Autodesk Inventor part; units mm, degrees
ref_plane "YZ Plane" through (0, 0, 0) normal (1, 0, 0) x (0, 1, 0)
ref_plane "XZ Plane" through (0, 0, 0) normal (0, 1, 0) x (-1, 0, 0)
ref_plane "XY Plane" through (0, 0, 0) normal (0, 0, 1) x (1, 0, 0)
sketch "Sketch1" plane through (0, 0, 0) normal (0, 1, 0) x (-1, 0, 0)
  line L0 (-27.5, 44) -> (27.5, 44)
  line L1 (27.5, 44) -> (27.5, -44)
  line L2 (27.5, -44) -> (-27.5, -44)
  line L3 (-27.5, -44) -> (-27.5, 44)
  line L4 (-27.5, 44) -> (27.5, -44) construction
  line L5 (27.5, 44) -> (-27.5, -44) construction
  line L6 (-27.5, 44) -> (-22.5, 44)
  line L7 (-22.5, 44) -> (-22.5, 35)
  line L8 (-22.5, 35) -> (-27.5, 35)
  line L9 (-27.5, 35) -> (-27.5, 44)
  line L10 (-22.5, 35) -> (-17.5, 35)
  line L11 (-17.5, 35) -> (-17.5, 30)
  line L12 (-17.5, 30) -> (-22.5, 30)
  line L13 (-22.5, 30) -> (-22.5, 35)
  line L14 (-17.5, 30) -> (-12.5, 30)
  line L15 (-12.5, 30) -> (-12.5, 25)
  line L16 (-12.5, 25) -> (-17.5, 25)
  line L17 (-17.5, 25) -> (-17.5, 30)
  line L18 (-12.5, 25) -> (-7.5, 25)
  line L19 (-7.5, 25) -> (-7.5, 20)
  line L20 (-7.5, 20) -> (-12.5, 20)
  line L21 (-12.5, 20) -> (-12.5, 25)
  line L22 (-7.5, 20) -> (-2.5, 20)
  line L23 (-2.5, 20) -> (-2.5, 15)
  line L24 (-2.5, 15) -> (-7.5, 15)
  line L25 (-7.5, 15) -> (-7.5, 20)
  line L26 (-2.5, 15) -> (2.5, 15)
  line L27 (2.5, 15) -> (2.5, 10)
  line L28 (2.5, 10) -> (-2.5, 10)
  line L29 (-2.5, 10) -> (-2.5, 15)
  line L30 (2.5, 10) -> (7.5, 10)
  line L31 (7.5, 10) -> (7.5, 5)
  line L32 (7.5, 5) -> (2.5, 5)
  line L33 (2.5, 5) -> (2.5, 10)
  line L34 (13, 5) -> (13, 0)
  line L35 (13, 0) -> (8, 0)
  line L36 (8, 0) -> (8, 5)
  line L37 (-27.5, -44) -> (27.5, 44) construction
  line L38 (-22.5, -35) -> (-27.5, -35)
  line L39 (-17.5, -30) -> (-22.5, -30)
  line L40 (-22.5, -30) -> (-22.5, -35)
  line L41 (-17.5, -25) -> (-17.5, -30)
  line L42 (-7.5, -20) -> (-12.5, -20)
  line L43 (-12.5, -20) -> (-12.5, -25)
  line L44 (-2.5, -15) -> (-7.5, -15)
  line L45 (-7.5, -15) -> (-7.5, -20)
  line L46 (2.5, -10) -> (-2.5, -10)
  line L47 (-2.5, -10) -> (-2.5, -15)
  line L48 (7.5, -5) -> (2.5, -5)
  line L49 (2.5, -5) -> (2.5, -10)
  line L50 (8, 0) -> (8, -5)
  line L51 (7.5, 5) -> (7.5, -5)
  line L52 (27.5, 0) -> (21.5, 0)
  circle A0 centre (21.5, 0) radius 6
  line L53 (-12.5, -25) -> (-17.5, -25)
  point P0 (0, 0)
  dimension "d0" = 55
  dimension "d1" = 88
  dimension "d2" = 5
  dimension "d3" = 9
  dimension "d4" = 5
  dimension "d5" = 5
  dimension "d6" = 5
  dimension "d7" = 5
  dimension "d8" = 5
  dimension "d9" = 5
  dimension "d10" = 5
  dimension "d11" = 5
  dimension "d12" = 5
  dimension "d13" = 5
  dimension "d14" = 5
  dimension "d15" = 5
  dimension "d16" = 5
  dimension "d17" = 5
  dimension "d18" = 6
extrude "Extrusion1" add sketch "Sketch1" along normal blind 20 contours L0 L7 L8 L3 | A0 | L0 L1 L2 L3 L38 L40 L39 L41 L53 L43 L42 L45 L44 L47 L46 L49 L48 L51 L31 L30 L27 L26 L23 L22 L19 L18 L15 L14 L11 L10 L7 | L10 L11 L12 L13 | L14 L15 L16 L17 | L18 L19 L20 L21 | L22 L23 L24 L25 | L26 L27 L28 L29 | L30 L31 L32 L33
sketch "Sketch2" plane through (0, 0, 0) normal (0, -1, 0) x (1, 0, 0)
  line L0 (-27.5, -44) -> (-27.5, 44)
  line L1 (-27.5, 0) -> (-21.5, 0)
  circle A0 centre (-21.5, 0) radius 6
  line L2 (-21.5, -6) -> (-27.5, -6)
  line L3 (-21.5, 6) -> (-27.5, 6)
  point P0 (0, 0)
  dimension "d21" = 6
extrude "Extrusion2" add sketch "Sketch2" along normal blind 11
sketch "Sketch3" plane through (0, 20, 0) normal (0, 1, 0) x (1, 0, 0)
  line L0 (-21.5, -6) -> (-27.5, -6)
  line L1 (-27.5, -6) -> (-27.5, 6)
  line L2 (-27.5, 6) -> (-21.5, 6)
  arc A0 (-21.5, -6) -> (-21.5, 6) centre (-21.5, 0) ccw
  point P0 (0, 0)
extrude "Extrusion3" add sketch "Sketch3" along normal blind 11
sketch "Sketch4" plane through (0, 31, 0) normal (0, 1, 0) x (1, 0, 0)
  arc A0 (-21.5, -6) -> (-21.5, 6) centre (-21.5, 0) ccw
  circle A1 centre (-21.5, 0) radius 2
  point P0 (0, 0)
  dimension "d26" = 4
extrude "Extrusion4" cut sketch "Sketch4" against normal through all
sketch "Sketch5" plane through (-27.5, 0, 44) normal (-1, 0, 0) x (0, 0, 1)
  line L0 (-44, 0) -> (-44, 10)
  line L1 (-46, 31) -> (-46, -11)
hole "Hole1" at (-27.5, 10, 0) direction (1, 0, 0) diameter 16 depth 10 tip angle 118
sketch "Sketch6" plane through (-27.5, 0, 44) normal (-1, 0, 0) x (0, 0, 1)
  line L0 (1.5, 16) -> (-1.5, 16)
  line L1 (-1.5, 16) -> (-1.5, 4)
  line L2 (-1.5, 4) -> (1.5, 4)
  line L3 (1.5, 4) -> (1.5, 16)
  line L4 (0, 0) -> (0, 20)
  line L5 (1.5, 16) -> (-1.5, 4) construction
  line L6 (-1.5, 16) -> (1.5, 4) construction
  line L7 (-89.5, 16) -> (-86.5, 16)
  line L8 (-86.5, 16) -> (-86.5, 4)
  line L9 (-86.5, 4) -> (-89.5, 4)
  line L10 (-89.5, 4) -> (-89.5, 16)
  line L11 (-88, 0) -> (-88, 20)
  line L12 (-89.5, 16) -> (-86.5, 4) construction
  line L13 (-86.5, 16) -> (-89.5, 4) construction
  point P0 (-44, 0)
  point P1 (0, 10)
  point P2 (-88, 10)
  dimension "d36" = 3
  dimension "d37" = 12
  dimension "d38" = 3
  dimension "d39" = 12
extrude "Extrusion5" cut sketch "Sketch6" against normal through all
fillet "Fillet1" radius 0.5 4 edges at (0, 4, 42.5) (0, 16, 42.5) (0, 4, -42.5) (0, 16, -42.5)
fillet "Fillet2" radius 1 6 edges at (-24.5, 20, -6) (-15.5, 20, 0) (-24.5, 20, 6) (-15.5, 0, 0) (-24.5, 0, 6) (-24.5, 0, -6)
chamfer "Chamfer1" distance 0.5 angle 45 8 edges at (0, 20, -44) (0, 16, -44) (0, 4, -44) (0, 0, -44) (0, 20, 44) (0, 16, 44) (0, 0, 44) (0, 4, 44)
thread "Thread1"
thread "Thread2"
properties part number "pfa"
Verification items for the finished model (mm, model axes). A direction names the side the tool comes from. Give positions to 0.01 mm unless a question says otherwise; leave off trailing zeros. Write each loop counter-clockwise with the first axis right and the second up, starting at its lowest first coordinate (ties: lowest second). Pieces come first, ordered by that corner, then holes. Notation, with made-up numbers: M -26,37 L -19,37 A16 cw -19,45 Z; hole C -13,68 d6. An arc over 180 degrees is marked long. Write item = value, one per line.
(1) Material ranges on line 1 (Z direction, x = -23.5, y = 10); line 2 (Z direction, x = -2, y = 14.5); line 3 (X direction, y = 25, z = 0), recorded low to high.
Found:
line_1 = -42.5 to -8, 8 to 42.5
line_2 = -42.5 to -10, 10 to 42.5
line_3 = -27.5 to -23.5, -19.5 to -15.5
(2) Go/stop test with flat-tipped pins: pin 1 Ø6.5 at (x, y) = (-24.5, 28.5) entering from -Z; pin 2 Ø4 at (x, y) = (5, 9.5) entering from +Z; pin 3 Ø1.5 at (y, z) = (6, 17) entering from +X; pin 4 Ø6 at (x, y) = (16.5, -3.5) entering from +Z. Record where each tip stops, or that it passes through.
Found:
pin_1 = -6
pin_2 = 42.5
pin_3 = 7.5
pin_4 = through
(3) Sectioned sample at B-B (y = 28). Record the cut outline in (x, z).
Found:
outline = M -27.5,-6 L -21.5,-6 A6 ccw -21.5,6 L -27.5,6 Z; hole C -21.5,0 d4
(4) Sectioned sample at A-A (x = 19.5). Record the cut outline in (y, z).
Found:
outline = M 0,-43.5 L 0.5,-44 L 3.5,-44 L 4,-43.5 L 4,-43 A0.5 cw 4.5,-42.5 L 15.5,-42.5 A0.5 cw 16,-43 L 16,-43.5 L 16.5,-44 L 19.5,-44 L 20,-43.5 L 20,-30 L 0,-30 Z; M 0,30 L 20,30 L 20,43.5 L 19.5,44 L 16.5,44 L 16,43.5 L 16,43 A0.5 cw 15.5,42.5 L 4.5,42.5 A0.5 cw 4,43 L 4,43.5 L 3.5,44 L 0.5,44 L 0,43.5 Z
(5) Draft check along Z on faces 4 (the face through (-25, 26, -6)), 5 (the face through (-24, -6, 6)), 6 (the face through (15, 10, 25)). Enter one of: released by +Z, released by -Z, zero draft, split by the parting line, or undercut.
Found:
face_4 = released by -Z
face_5 = released by +Z
face_6 = undercut
(6) Sectioned sample at C-C (z = 28). Record the cut outline in (x, y), then the cut area to 3 significant figures.
Found:
outline = M -27.5,0 L 17.5,0 L 17.5,20 L -27.5,20 Z
area = 900 mm2
(7) Access from +Z, -Z, +X, -X, +Y, -Y to the whole of each face (thin tool, end or side, straight path). Record for faces 1 (the face through (7.5, 10, 17)), 2 (the face through (-15.5, 25.9, -0.1)), 3 (the face through (0, 2, 44)).
Found:
face_1 = +X, +Y, -Y
face_2 = +X, +Y
face_3 = +Z, +X, -X, +Y, -Y
(8) Sectioned sample at D-D (z = -12.5). Record the cut outline in (x, y).
Found:
outline = M -27.5,0 L 2.5,0 L 2.5,20 L -27.5,20 Z
